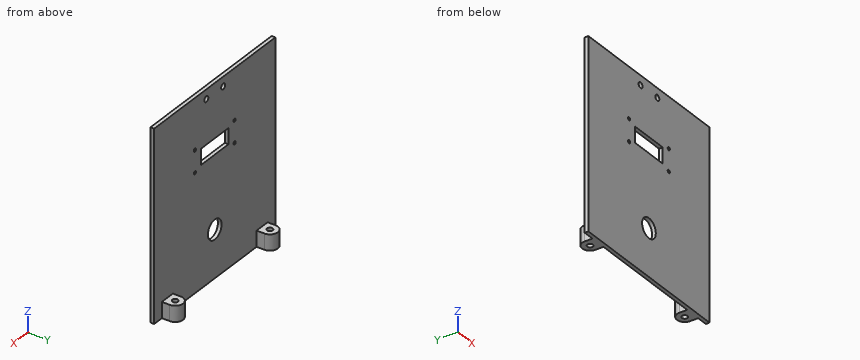
```python
from build123d import *

# Parameters (mm, degrees)
SKETCH1_W               = 139.5
SKETCH1_H               = 152.4
BOSS_EXTRUDE1_DEPTH     = 6.35
SKETCH2_W               = 139.5
SKETCH2_H               = 152.4
CUT_EXTRUDE1_DEPTH      = 3.375
SKETCH4_R               = 2.286
BOSS_EXTRUDE3_DEPTH     = 12.7
SKETCH5_R               = 7.874
CUT_EXTRUDE2_DEPTH      = 16.675
SKETCH6_R               = 2.286
CUT_EXTRUDE3_DEPTH      = 3.975
SKETCH7_R               = 1.27
SKETCH7_W               = 31.75
SKETCH7_H               = 12.7
CUT_EXTRUDE4_DEPTH      = 1
CUT_EXTRUDE4_DEPTH_BACK = 16.675


with BuildPart() as part:
    # Sketch1 → Boss-Extrude1 (new body)
    with BuildSketch(Plane(origin=(0, 0, 0), x_dir=(1, 0, 0), z_dir=(0, 1, 0))):
        with Locations((69.75, 76.2)):
            Rectangle(SKETCH1_W, SKETCH1_H)
    extrude(amount=BOSS_EXTRUDE1_DEPTH)

    # Sketch2 → Cut-Extrude1 (cut)
    with BuildSketch(Plane(origin=(0, 6.35, 0), x_dir=(1, 0, 0), z_dir=(0, 1, 0))):
        with Locations((69.75, 76.2)):
            Rectangle(SKETCH2_W, SKETCH2_H)
    extrude(amount=-CUT_EXTRUDE1_DEPTH, mode=Mode.SUBTRACT)

    # Sketch4 → Boss-Extrude3 (add)
    with BuildSketch(Plane(origin=(0, 0, -152.4), x_dir=(-1, 0, 0), z_dir=(0, 0, -1))):
        with BuildLine():
            Line((-130.61, 9.325), (-130.61, 2.975))
            Line((-130.61, 2.975), (-117.91, 2.975))
            Line((-117.91, 2.975), (-117.91, 9.325))
            ThreePointArc((-117.91, 9.325), (-124.26, 15.675), (-130.61, 9.325))
        make_face()
        with Locations((-124.26, 9.325)):
            Circle(SKETCH4_R, mode=Mode.SUBTRACT)
        with BuildLine():
            Line((-21.59, 9.325), (-21.59, 2.975))
            Line((-21.59, 2.975), (-8.89, 2.975))
            Line((-8.89, 2.975), (-8.89, 9.325))
            ThreePointArc((-8.89, 9.325), (-15.24, 15.675), (-21.59, 9.325))
        make_face()
        with Locations((-15.24, 9.325)):
            Circle(SKETCH4_R, mode=Mode.SUBTRACT)
    extrude(amount=-BOSS_EXTRUDE3_DEPTH)

    # Sketch5 → Cut-Extrude2 (cut, through all)
    with BuildSketch(Plane.XZ):
        with Locations((69.75, -114.3)):
            Circle(SKETCH5_R)
    extrude(amount=-CUT_EXTRUDE2_DEPTH, mode=Mode.SUBTRACT)

    # Sketch6 → Cut-Extrude3 (cut, through all)
    with BuildSketch(Plane(origin=(0, 2.975, 0), x_dir=(1, 0, 0), z_dir=(0, 1, 0))):
        with Locations((60.098, 7.62)):
            Circle(SKETCH6_R)
        with Locations((79.402, 7.62)):
            Circle(SKETCH6_R)
    extrude(amount=-CUT_EXTRUDE3_DEPTH, mode=Mode.SUBTRACT)

    # Sketch7 → Cut-Extrude4 (cut, two sides)
    with BuildSketch(Plane.XZ) as cut_extrude4_sk:
        with Locations((46.89, -40.64)):
            Circle(SKETCH7_R)
        with Locations((92.61, -40.64)):
            Circle(SKETCH7_R)
        with Locations((92.61, -58.42)):
            Circle(SKETCH7_R)
        with Locations((46.89, -58.42)):
            Circle(SKETCH7_R)
        with Locations((69.75, -49.53)):
            Rectangle(SKETCH7_W, SKETCH7_H)
    extrude(amount=CUT_EXTRUDE4_DEPTH, mode=Mode.SUBTRACT)
    extrude(cut_extrude4_sk.sketch, amount=-CUT_EXTRUDE4_DEPTH_BACK, mode=Mode.SUBTRACT)


solid = part.part
```
CAD build for the part. Positions are in the model's coordinates, mm. Round coordinates to 2 decimals unless told otherwise and drop trailing zeros. Write each loop counter-clockwise with the first axis right and the second up, starting at its lowest first coordinate (ties: lowest second). Pieces come first, ordered by that corner, then holes. Notation, with made-up numbers: (-18.5, 40) -> (20.5, 40) arc R22 cw to (20.5, 77) -> close; hole circle Ø6 at (78.5, -30). An arc over 180 degrees is marked (long way). Answer in a Markdown table with one row per item. Add a question column.
Item 1: Drop flat-ended pins along their axis: pin 1 Ø6.5 at (x, y) = (17, 6.5) entering from +Z; pin 2 Ø4 at (x, z) = (45.5, -111) entering from +Y (3 decimals); pin 3 Ø7 at (y, z) = (7, -145) entering from +X. Give the stop position or say it passes through.
Item 2: Saw through at A-A, the plane x = 69.75. Write the cut outline in (y, z) (3 decimals), then the cut area to 3 significant figures.
Item 3: Saw through at B-B, the plane z = -114.3. Write the cut outline in (x, y) (3 decimals), then the cut area to 3 significant figures.
Item 4: Saw through at D-D, the plane x = 99. Write the cut outline in (y, z) (3 decimals).
Item 5: Saw through at C-C, the plane z = -142. Write the cut outline in (x, y) (3 decimals).
Item 6: Drill centre lines: line 1 (Z direction, x = 92.61, y = 0.8); line 2 (X direction, y = 1.9, z = -7.62); line 3 (X direction, y = 5.25, z = -145.5). Where is each one in solid material? Low to high. Write a range as from..to.
Findings below:
| question | item | result |
|---|---|---|
| 1 | pin 1 | stops at z = -139.7 |
| 1 | pin 2 | stops at y = 2.975 |
| 1 | pin 3 | stops at x = 130.61 |
| 2 | outline | (0, -152.4) -> (2.975, -152.4) -> (2.975, -122.174) -> (0, -122.174) -> close; (0, -106.426) -> (2.975, -106.426) -> (2.975, -55.88) -> (0, -55.88) -> close; (0, -43.18) -> (2.975, -43.18) -> (2.975, 0) -> (0, 0) -> close |
| 2 | area | 369 mm^2 |
| 3 | outline | (0, 0) -> (61.876, 0) -> (61.876, 2.975) -> (0, 2.975) -> close; (77.624, 0) -> (139.5, 0) -> (139.5, 2.975) -> (77.624, 2.975) -> close |
| 3 | area | 368 mm^2 |
| 4 | outline | (0, -152.4) -> (2.975, -152.4) -> (2.975, 0) -> (0, 0) -> close |
| 5 | outline | (0, 0) -> (139.5, 0) -> (139.5, 2.975) -> (130.61, 2.975) -> (130.61, 9.325) arc R6.35 ccw to (117.91, 9.325) -> (117.91, 2.975) -> (21.59, 2.975) -> (21.59, 9.325) arc R6.35 ccw to (8.89, 9.325) -> (8.89, 2.975) -> (0, 2.975) -> close; hole circle Ø4.572 at (15.24, 9.325); hole circle Ø4.572 at (124.26, 9.325) |
| 6 | line 1 | z = -152.4..-59.69, -57.15..-41.91, -39.37..0 |
| 6 | line 2 | x = 0..57.81, 62.38..77.12, 81.69..139.5 |
| 6 | line 3 | x = 8.89..21.59, 117.91..130.61 |
